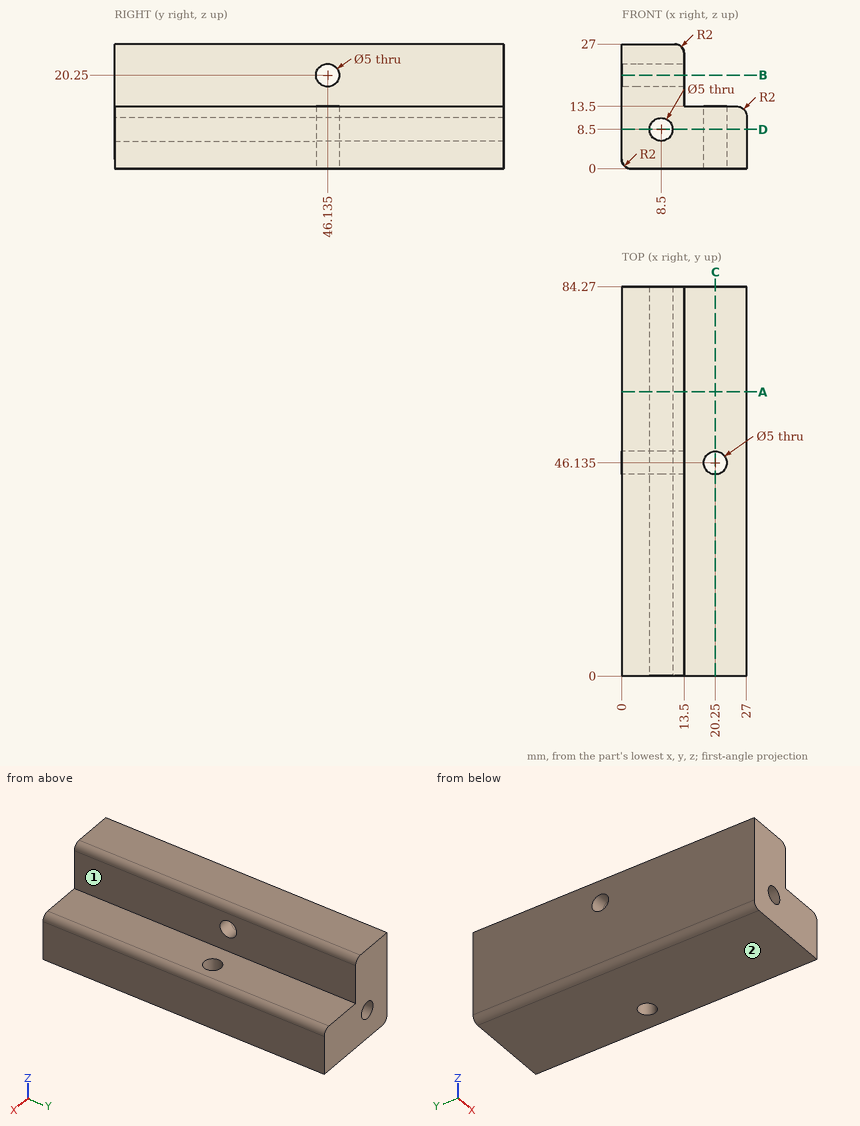
The drawing under review shows one solid part. Ordinate dimensions are in mm from its lowest x, y, z. A direction names the side the tool comes from. Coordinates: 2 decimals unless noted, no trailing zeros. Write each loop counter-clockwise with the first axis right and the second up, starting at its lowest first coordinate (ties: lowest second). Pieces come first, ordered by that corner, then holes. Notation, with made-up numbers: (-11.75, 71) - (14.25, 71) arc R21 cw to (14.25, 96) - close; hole circle Ø1 at (-40, 72.25). An arc over 180 degrees is marked (long way). Answer as CSV lines item,"result".
(1) We need section C-C (x = 20.25). Give the boundary of the cut face in (y, z) (3 decimals).
Data:
outline,"(0, 0) - (43.635, 0) - (43.635, 13.5) - (0, 13.5) - close; (48.635, 0) - (84.27, 0) - (84.27, 13.5) - (48.635, 13.5) - close"
(2) We need section D-D (z = 8.5). Give the boundary of the cut face in (x, y) (3 decimals), plus the area to 3 significant figures.
Data:
outline,"(0, 0) - (6, 0) - (6, 84.27) - (0, 84.27) - close; (11, 0) - (27, 0) - (27, 84.27) - (11, 84.27) - close; hole circle Ø5 at (20.25, 46.135)"
area,"1,830 mm2"
(3) Clearance check with flat-ended pins moving along their axes: pin 1 Ø3.5 at (y, z) = (30, 20) entering from +X; pin 2 Ø10 at (y, z) = (32.5, 17) entering from +X; pin 3 Ø3.5 at (x, y) = (21, 40.5) entering from +Z; pin 4 Ø1.5 at (x, y) = (20, 18) entering from -Z. State where each tip first meets the part, or that it passes through.
Data:
pin 1,"stops at x = 13.5"
pin 2,"stops at x = 26.94"
pin 3,"stops at z = 13.5"
pin 4,"stops at z = 0"
(4) For line 1 along X through (y, z) = (62.5, 8.5); line 2 along Y through (x, z) = (5.5, 20.25) (3 decimals); line 3 along X through (y, z) = (56, 11.75), list the stretches that pass through material, from the lowest coordinate up. Write a range as [from, to].
Data:
line 1,"x = [0, 6], [11, 27]"
line 2,"y = [0, 43.635], [48.635, 84.27]"
line 3,"x = [0, 26.98]"
(5) We need section A-A (y = 61.5). Give the boundary of the cut face in (x, z), plus the area to 3 significant figures.
Data:
outline,"(0, 2) arc R2 ccw to (2, 0) - (27, 0) - (27, 11.5) arc R2 ccw to (25, 13.5) - (13.5, 13.5) - (13.5, 25) arc R2 ccw to (11.5, 27) - (0, 27) - close; hole circle Ø5 at (8.5, 8.5)"
area,"525 mm2"
(6) Tool access review of the marked faces 1 and 2: name each direction out of +Z, -Z, +X, -X, +Y, -Y from which nothing blocks a thin tool from reaching the whole face with its end or side.
Data:
face 1,"+Z, +X, +Y, -Y"
face 2,"-Z, +X, -X, +Y, -Y"
(7) We need section B-B (z = 20.25). Give the boundary of the cut face in (x, y) (3 decimals), plus the area to 3 significant figures.
Data:
outline,"(0, 0) - (13.5, 0) - (13.5, 43.635) - (0, 43.635) - close; (0, 48.635) - (13.5, 48.635) - (13.5, 84.27) - (0, 84.27) - close"
area,"1,070 mm2"
